Geometry: see drawing. Coordinates: mm, zero at the bounding-box minimum. A direction names the side the tool comes from. Round coordinates to 2 decimals unless told otherwise and drop trailing zeros. Order: outer loops, then holes, each group sorted by start corner. A loop starts at its lowest first (then second) coordinate and runs counter-clockwise, first axis right, second up. Notation, with made-up numbers: (-35.5, -33) -> (-0.5, -33) arc R31 cw to (-0.5, 4) -> close; hole circle Ø8 at (26, -27.5). An arc over 180 degrees is marked (long way). Put each result on its own line as item: value.
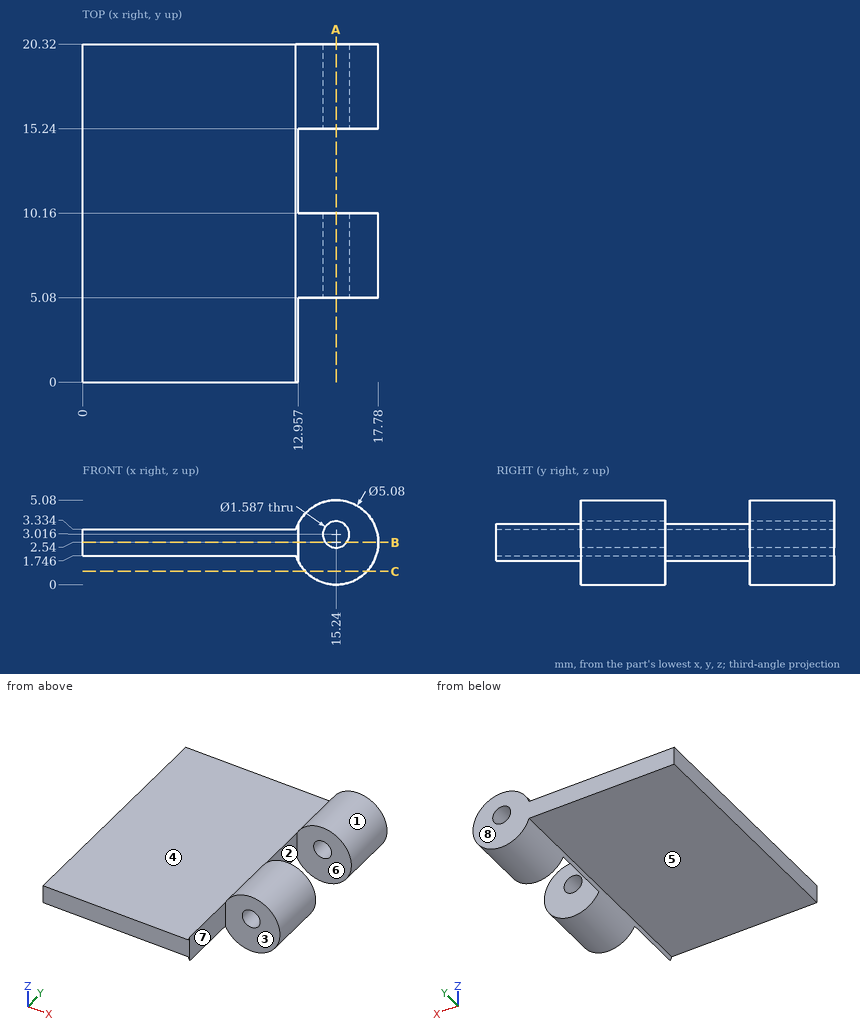
1. Cut plane C-C on z = 0.8. Return loops of the section in (x, y), and give its area (3 significant figures).
Ans:
outline: (13.39, 5.08) -> (17.09, 5.08) -> (17.09, 10.16) -> (13.39, 10.16) -> close; (13.39, 15.24) -> (17.09, 15.24) -> (17.09, 20.32) -> (13.39, 20.32) -> close
area: 37.6 mm²
2. Contact query for flat-ended pins moving along their axis: P1, Ø8, axis at x = 3.5, y = 2, coming from the +Z side; P2, Ø2.5, axis at y = 13, z = 2.5, coming from the +X side; P3, Ø8, axis at x = 9.5, y = 16.5, coming from the +Z side. Output: stop coordinate, or through.
Ans:
P1: z = 3.33
P2: x = 12.96
P3: z = 4.39
3. Cut plane A-A on x = 15.24. Return loops of the section in (y, z).
Ans:
outline: (5.08, 0) -> (10.16, 0) -> (10.16, 2.22) -> (5.08, 2.22) -> close; (5.08, 3.81) -> (10.16, 3.81) -> (10.16, 5.08) -> (5.08, 5.08) -> close; (15.24, 0) -> (20.32, 0) -> (20.32, 2.22) -> (15.24, 2.22) -> close; (15.24, 3.81) -> (20.32, 3.81) -> (20.32, 5.08) -> (15.24, 5.08) -> close
4. Cut plane B-B on z = 2.54. Return loops of the section in (x, y) (1 decimal), and give its area (3 significant figures).
Ans:
outline: (0, 0) -> (13, 0) -> (13, 5.1) -> (14.6, 5.1) -> (14.6, 10.2) -> (13, 10.2) -> (13, 15.2) -> (14.6, 15.2) -> (14.6, 20.3) -> (0, 20.3) -> close; (15.9, 5.1) -> (17.8, 5.1) -> (17.8, 10.2) -> (15.9, 10.2) -> close; (15.9, 15.2) -> (17.8, 15.2) -> (17.8, 20.3) -> (15.9, 20.3) -> close
area: 299 mm²
5. Set-up query: the marked faces 4, 5, 6, 7 and 8. Return all of +Z, -Z, +X, -X, +Y, -Y with unobstructed straight access to the full face (end or side cutting, diameter ignored); none if empty.
Ans:
face 4: +Z, -X, +Y, -Y
face 5: -Z, -X, +Y, -Y
face 6: +Z, -Z, +X
face 7: +Z, -Z, +X, -Y
face 8: +Z, -Z, +X, -X, +Y
6. Draft query along Y for the marked faces 1, 2 and 3. Return one class per face: +Y half, -Y half, draft (parallel to the pull), parting line (faces both ways), or undercut.
Ans:
face 1: draft
face 2: undercut
face 3: -Y half
7. Material intervals for probe 1 along Y at (x, z) = (15.5, 0.4); probe 2 along Z at (x, y) = (10.5, 5.25); probe 3 along Z at (x, y) = (15.24, 9.1), sorted ascending.
Ans:
probe 1: 5.08 to 10.16, 15.24 to 20.32
probe 2: 1.75 to 3.33
probe 3: 0 to 2.22, 3.81 to 5.08
